Input: part model. Units: mm. Frame: model coordinates. A direction names the side the tool comes from. Give positions to 0.01 mm unless a question says otherwise; leave off trailing zeros. Loops run counter-clockwise (first coordinate to the right, second up) from the corner with the lowest first, then second, coordinate; pieces in that order, holes last. Notation, with made-up numbers: (-10.75, 7.5) - (6.25, 7.5) arc R20 ccw to (6.25, 20.5) - close; hole circle Ø10 at (-34.5, 43). An arc over 180 degrees is marked (long way). One line per item, written item: value.
from build123d import *

# Parameters (mm, degrees)
SKETCH_1_W               = 180
SKETCH_1_H               = 180
EXTRUDE_1_DEPTH          = 5
SKETCH_2_R               = 5.25
CUT_EXTRUDE_1_DEPTH      = 128.377392029
MIRROR_2_COPY_1_SKETCH_R = 5.25
MIRROR_2_COPY_1_DEPTH    = 128.377392029
SKETCH_3_W               = 87
SKETCH_3_H               = 87
SKETCH_3_W_2             = 81
SKETCH_3_H_2             = 81
EXTRUDE_2_DEPTH          = 150
EXTRUDE_3_DEPTH          = 2.5
EXTRUDE_4_DEPTH          = 2.5
CUT_EXTRUDE_2_DEPTH      = 224.488814038
MIRROR_6_COPY_1_DEPTH    = 224.488814038


with BuildPart() as part:
    # 草图1 → 凸台-拉伸1 (new body)
    with BuildSketch(Plane.XY):
        Rectangle(SKETCH_1_W, SKETCH_1_H)
    extrude(amount=EXTRUDE_1_DEPTH)

    # 草图2 → 切除-拉伸1 (cut, through all)
    with BuildSketch(Plane.XY.offset(5)):
        with Locations((-67.776804162, 69.299878413)):
            Circle(SKETCH_2_R)
    cut_extrude_1 = extrude(amount=-CUT_EXTRUDE_1_DEPTH, mode=Mode.SUBTRACT)

    # 镜向1: 切除-拉伸1 across plane
    add(cut_extrude_1.mirror(Plane.ZX), mode=Mode.SUBTRACT)

    # 镜向2: 切除-拉伸1 across plane
    add(cut_extrude_1.mirror(Plane(origin=(0, 0, 0), x_dir=(0, 0, 1), z_dir=(1, 0, 0))), mode=Mode.SUBTRACT)

    # 镜向2 copy 1 sketch → 镜向2 copy 1 (cut, through all)
    with BuildSketch(Plane(origin=(0, 0, 5), x_dir=(-1, 0, 0), z_dir=(0, 0, 1))):
        with Locations((-67.776804162, 69.299878413)):
            Circle(MIRROR_2_COPY_1_SKETCH_R)
    extrude(amount=-MIRROR_2_COPY_1_DEPTH, mode=Mode.SUBTRACT)

    # 草图3 → 凸台-拉伸2 (add)
    with BuildSketch(Plane.XY.offset(5)):
        Rectangle(SKETCH_3_W, SKETCH_3_H)
        Rectangle(SKETCH_3_W_2, SKETCH_3_H_2, mode=Mode.SUBTRACT)
    extrude(amount=EXTRUDE_2_DEPTH)

    # 草图4 → 凸台-拉伸3 (add, symmetric)
    with BuildSketch(Plane(origin=(0, 0, 0), x_dir=(1, 0, 0), z_dir=(0, 1, 0))):
        Polygon((43.5, -5), (90, -5), (43.5, -85), align=None)
    extrude_3 = extrude(amount=EXTRUDE_3_DEPTH, both=True)

    # 镜向3: 凸台-拉伸3 across plane
    add(extrude_3.mirror(Plane(origin=(0, 0, 0), x_dir=(0, 0, 1), z_dir=(1, 0, 0))))

    # 草图5 → 凸台-拉伸4 (add, symmetric)
    with BuildSketch(Plane(origin=(0, 0, 0), x_dir=(0, 0, -1), z_dir=(1, 0, 0))):
        Polygon((-5, 43.5), (-5, 90), (-85, 43.5), align=None)
    extrude_4 = extrude(amount=EXTRUDE_4_DEPTH, both=True)

    # 镜向4: 凸台-拉伸4 across plane
    add(extrude_4.mirror(Plane.ZX))

    # 草图6 → 切除-拉伸2 (cut, through all)
    with BuildSketch(Plane.XZ.offset(43.5)):
        with BuildLine():
            Line((-14.50686738, 121.547822852), (-14.50686738, 110.547822852))
            ThreePointArc((-14.50686738, 110.547822852), (-19.00686738, 106.047822852), (-23.50686738, 110.547822852))
            Line((-23.50686738, 110.547822852), (-23.50686738, 121.547822852))
            ThreePointArc((-23.50686738, 121.547822852), (-19.00686738, 126.047822852), (-14.50686738, 121.547822852))
        make_face()
        with BuildLine():
            Line((-14.50686738, 56.214536174), (-14.50686738, 45.214536174))
            ThreePointArc((-14.50686738, 45.214536174), (-19.00686738, 40.714536174), (-23.50686738, 45.214536174))
            Line((-23.50686738, 45.214536174), (-23.50686738, 56.214536174))
            ThreePointArc((-23.50686738, 56.214536174), (-19.00686738, 60.714536174), (-14.50686738, 56.214536174))
        make_face()
    cut_extrude_2 = extrude(amount=-CUT_EXTRUDE_2_DEPTH, mode=Mode.SUBTRACT)

    # 镜向5: 切除-拉伸2 across plane
    add(cut_extrude_2.mirror(Plane(origin=(0, 0, 0), x_dir=(0, 0, 1), z_dir=(1, 0, 0))), mode=Mode.SUBTRACT)

    # 镜向6: 切除-拉伸2 across plane
    add(cut_extrude_2.mirror(Plane(origin=(0, 0, 0), x_dir=(0, 0, 1), z_dir=(0.7071067811865483, -0.7071067811865468, 0))), mode=Mode.SUBTRACT)

    # 镜向6 copy 1 sketch → 镜向6 copy 1 (cut, through all)
    with BuildSketch(Plane(origin=(-43.5, 0, 0), x_dir=(0, -1, 0), z_dir=(-1, 0, 0))):
        with BuildLine():
            Line((-14.50686738, 121.547822852), (-14.50686738, 110.547822852))
            ThreePointArc((-14.50686738, 110.547822852), (-19.00686738, 106.047822852), (-23.50686738, 110.547822852))
            Line((-23.50686738, 110.547822852), (-23.50686738, 121.547822852))
            ThreePointArc((-23.50686738, 121.547822852), (-19.00686738, 126.047822852), (-14.50686738, 121.547822852))
        make_face()
        with BuildLine():
            Line((-14.50686738, 56.214536174), (-14.50686738, 45.214536174))
            ThreePointArc((-14.50686738, 45.214536174), (-19.00686738, 40.714536174), (-23.50686738, 45.214536174))
            Line((-23.50686738, 45.214536174), (-23.50686738, 56.214536174))
            ThreePointArc((-23.50686738, 56.214536174), (-19.00686738, 60.714536174), (-14.50686738, 56.214536174))
        make_face()
    extrude(amount=-MIRROR_6_COPY_1_DEPTH, mode=Mode.SUBTRACT)


solid = part.part
Item 1: Section C-C, the plane x = -65. Output: boundary loops of the cut face in (y, z), and give its area (3 significant figures).
Verdict:
outline: (-90, 0) - (-73.76, 0) - (-73.76, 5) - (-90, 5) - close; (-64.84, 0) - (64.84, 0) - (64.84, 5) - (2.5, 5) - (2.5, 48.01) - (-2.5, 48.01) - (-2.5, 5) - (-64.84, 5) - close; (73.76, 0) - (90, 0) - (90, 5) - (73.76, 5) - close
area: 1,030 mm^2
Item 2: Draft query along X for faces 4 (the face through (-18.91, 41.98, 106.05)), 5 (the face through (-1, 1, 0)), 6 (the face through (43.5, 9, 79)), 7 (the face through (18.91, -42.02, 106.05)). Return one class per face: pulls with the +X half, pulls with the -X half, needs draft (parallel to the pull), parting line crosses it, or undercut.
Verdict:
face 4: undercut
face 5: needs draft
face 6: pulls with the +X half
face 7: undercut
Item 3: Access query for faces 1 (the face through (-19.106, -42.021, 60.713)), 2 (the face through (41.979, 19.106, 60.713)), 3 (the face through (-43.5, 9, 79)). Directions: +Z, -Z, +X, -X, +Y, -Y. A direction counts if a zero-diameter tool reaches every point of the face in a straight line with its end or side. Return the directions, or none.
Verdict:
face 1: +Y, -Y
face 2: +X, -X
face 3: +Z, -X
Item 4: Section B-B, the plane y = 29. Output: boundary loops of the cut face in (x, z), and give its area (3 significant figures).
Verdict:
outline: (-90, 0) - (90, 0) - (90, 5) - (43.5, 5) - (43.5, 155) - (40.5, 155) - (40.5, 5) - (-40.5, 5) - (-40.5, 155) - (-43.5, 155) - (-43.5, 5) - (-90, 5) - close
area: 1,800 mm^2
Item 5: Section D-D, the plane z = 17.5. Output: boundary loops of the cut face in (x, y), and give its area (3 significant figures).
Verdict:
outline: (-82.73, -2.5) - (-43.5, -2.5) - (-43.5, -43.5) - (-2.5, -43.5) - (-2.5, -82.73) - (2.5, -82.73) - (2.5, -43.5) - (43.5, -43.5) - (43.5, -2.5) - (82.73, -2.5) - (82.73, 2.5) - (43.5, 2.5) - (43.5, 43.5) - (2.5, 43.5) - (2.5, 82.73) - (-2.5, 82.73) - (-2.5, 43.5) - (-43.5, 43.5) - (-43.5, 2.5) - (-82.73, 2.5) - close; hole (-40.5, -40.5) - (40.5, -40.5) - (40.5, 40.5) - (-40.5, 40.5) - close
area: 1,790 mm^2
Item 6: Section A-A, the plane z = 129. Output: boundary loops of the cut face in (x, y), and give its area (3 significant figures).
Verdict:
outline: (-43.5, -43.5) - (43.5, -43.5) - (43.5, 43.5) - (-43.5, 43.5) - close; hole (-40.5, -40.5) - (40.5, -40.5) - (40.5, 40.5) - (-40.5, 40.5) - close
area: 1,010 mm^2
Item 7: Pin query (flat end, axial travel): P1, Ø10, axis at x = -33.5, y = -65.5, coming from the +Z side; P2, Ø0.9, axis at x = 42, z = 49.5, coming from the -Y side; P3, Ø12, axis at y = 15, z = 94.5, coming from the -X side; P4, Ø5, axis at x = -60.5, y = -2.5, coming from the -Z side. Return the tip coordinate at first contact, or that it passes through.
Verdict:
P1: stops at z = 5
P2: stops at y = -43.5
P3: stops at x = -43.5
P4: stops at z = 0
Item 8: Material intervals for L1, parallel to Y at x = -23.5, z = 84; L2, parallel to Z at x = -68, y = -36.5, sorted ascending.
Verdict:
L1: y = -43.5 to -40.5, 40.5 to 43.5
L2: z = 0 to 5
